Drawing for the job (mm, zero at the part's lowest x, y, z). Give positions to 0.01 mm unless a question says otherwise; leave off trailing zeros. Order: outer loops, then holes, each group sorted by start corner. A loop starts at its lowest first (then second) coordinate and runs counter-clockwise, first axis right, second up. Notation, with made-up numbers: (56, -5.75) - (113, -5.75) arc R28 cw to (113, 29.25) - close; hole circle Ø11 at (11.5, -38.5). An arc over 180 degrees is marked (long way). One line per item, written item: value.
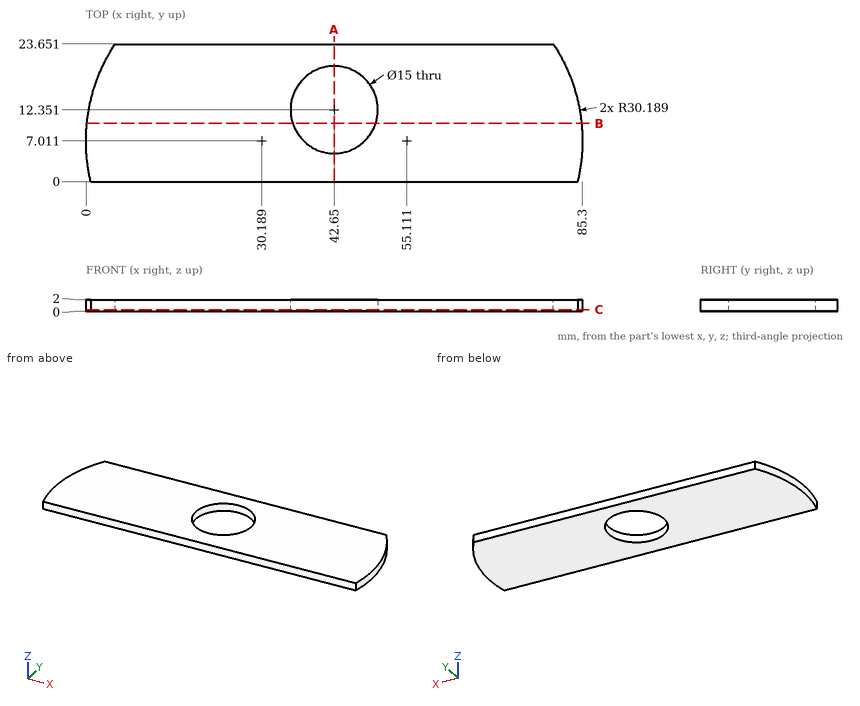
1) Pin check, flat tip, straight feed: pin 1 (1.5 mm diameter, centred on x = 50, y = 13.5, fed in from +Z). Stop position of the tip, or through.
Outcome:
pin 1: stops at z = 2
2) Cut at C-C, the plane z = 0.3. Give the cut face in (x, y), then the cut area to 3 significant figures.
Outcome:
outline: (0.83, 0) - (84.47, 0) arc R30.19 ccw to (80.3, 23.65) - (5, 23.65) arc R30.19 ccw to start; hole circle Ø15 at (42.65, 12.35)
area: 1,780 mm^2
3) Drill centre lines: line 1 along Y through (x, z) = (42.65, 1.35); line 2 along X through (y, z) = (7, 1.2) (1 decimal); line 3 along X through (y, z) = (14.5, 0.95) (1 decimal). Where is each one in solid material? Low to high. Write a range as from..to.
Outcome:
line 1: y = 0..4.85, 19.85..23.65
line 2: x = 0..37.4, 47.9..85.3
line 3: x = 0.9..35.5, 49.8..84.4
4) Cut at B-B, the plane y = 10. Give the cut face in (x, z).
Outcome:
outline: (0.15, 0) - (35.53, 0) - (35.53, 2) - (0.15, 2) - close; (49.77, 0) - (85.15, 0) - (85.15, 2) - (49.77, 2) - close
5) Cut at A-A, the plane x = 42.65. Give the cut face in (y, z), then the cut area to 3 significant figures.
Outcome:
outline: (0, 0) - (4.85, 0) - (4.85, 2) - (0, 2) - close; (19.85, 0) - (23.65, 0) - (23.65, 2) - (19.85, 2) - close
area: 17.3 mm^2
